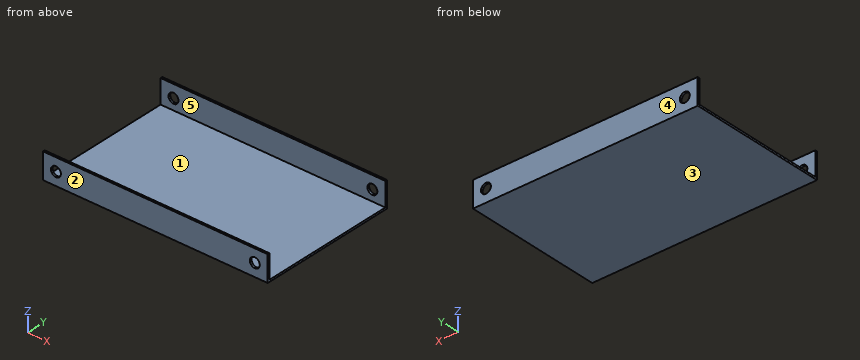
from build123d import *

# Parameters (mm, degrees)
SKETCH3_W               = 287.02
SKETCH3_H               = 177.8
BOSS_EXTRUDE1_DEPTH     = 33.02
SKETCH4_W               = 281.94
SKETCH4_H               = 172.72
CUT_EXTRUDE1_DEPTH      = 30.48
CUT_EXTRUDE2_DEPTH      = 300.87064011
CUT_EXTRUDE2_DEPTH_BACK = 300.87064011
SKETCH5_W               = 30.48
SKETCH5_H               = 172.72
CUT_EXTRUDE3_DEPTH      = 229.913756904
CUT_EXTRUDE3_DEPTH_BACK = 229.913756904
SKETCH6_R               = 6.35


with BuildPart() as part:
    # Sketch3 → Boss-Extrude1 (new body)
    with BuildSketch(Plane.XY):
        Rectangle(SKETCH3_W, SKETCH3_H)
    extrude(amount=BOSS_EXTRUDE1_DEPTH)

    # Sketch4 → Cut-Extrude1 (cut)
    with BuildSketch(Plane.XY.offset(33.02)):
        Rectangle(SKETCH4_W, SKETCH4_H)
    extrude(amount=-CUT_EXTRUDE1_DEPTH, mode=Mode.SUBTRACT)

    # Sketch5 → Cut-Extrude2 (cut, two sides: drawn at the far end of the back side and taken through both)
    with BuildSketch(Plane(origin=(-140.97, 0, 0), x_dir=(0, 0, -1), z_dir=(1, 0, 0)).offset(-CUT_EXTRUDE2_DEPTH_BACK)):
        with Locations((-17.78, 0)):
            Rectangle(SKETCH5_W, SKETCH5_H)
    extrude(amount=CUT_EXTRUDE2_DEPTH + CUT_EXTRUDE2_DEPTH_BACK, mode=Mode.SUBTRACT)

    # Sketch6 → Cut-Extrude3 (cut, two sides: drawn at the far end of the back side and taken through both)
    with BuildSketch(Plane(origin=(0, -86.36, 0), x_dir=(1, 0, 0), z_dir=(0, 1, 0)).offset(-CUT_EXTRUDE3_DEPTH_BACK)):
        with Locations(Location((127, -16.51, 0), (0, 0, 270))):
            Circle(SKETCH6_R)
        with Locations(Location((-127, -16.51, 0), (0, 0, 270))):
            Circle(SKETCH6_R)
    extrude(amount=CUT_EXTRUDE3_DEPTH + CUT_EXTRUDE3_DEPTH_BACK, mode=Mode.SUBTRACT)


solid = part.part
Check sheet for the modelled part. Datum: model origin and axes. Units: mm. Face numbers are marked on the shaded views. A direction names the side the tool comes from. Round coordinates to 2 decimals unless told otherwise and drop trailing zeros. Order: outer loops, then holes, each group sorted by start corner. A loop starts at its lowest first (then second) coordinate and runs counter-clockwise, first axis right, second up.
(1) Cross-section at D-D, the plane y = -61. Enter the section's corners in (x, z).
(2) Access from +Z, -Z, +X, -X, +Y, -Y to the whole of each face (thin tool, end or side, straight path). Record for the marked faces 4 and 5.
(3) Cross-section at B-B, the plane x = 127. Enter the section's corners in (y, z).
(4) Scan lines: probe 1 along X at (y, z) = (87, 16.51); probe 2 along Y at (x, z) = (85.5, 20); probe 3 along Z at (x, y) = (127, 88.35). Record each from-to range of solid material in increasing order.
(5) Cross-section at C-C, the plane x = -14.5. Enter the section's corners in (y, z), and give its area (3 significant figures).
(6) Draft check along Y on the marked faces 1, 2 and 3. Enter one of: pulls with the +Y half, pulls with the -Y half, needs draft (parallel to the pull), parting line crosses it, or undercut.
(7) Go/stop test with flat-tipped pins: P1, Ø1, axis at x = -85, y = -20, coming from the +Z side; P2, Ø11.5, axis at x = 127, z = 16.51, coming from the +Y side. Record where each tip stops, or that it passes through.
(8) Cross-section at A-A, the plane z = 27. Enter the section's corners in (x, y), and give its area (3 significant figures).
Check sheet entries:
1. outline: (-143.51, 0) - (143.51, 0) - (143.51, 2.54) - (-143.51, 2.54) - close
2. face 4: +Z, -Z, +X, -X, +Y
2. face 5: +Z, +X, -X
3. outline: (-88.9, 0) - (88.9, 0) - (88.9, 10.16) - (86.36, 10.16) - (86.36, 2.54) - (-86.36, 2.54) - (-86.36, 10.16) - (-88.9, 10.16) - close; (-88.9, 22.86) - (-86.36, 22.86) - (-86.36, 33.02) - (-88.9, 33.02) - close; (86.36, 22.86) - (88.9, 22.86) - (88.9, 33.02) - (86.36, 33.02) - close
4. probe 1: x = -143.51 to -133.35, -120.65 to 120.65, 133.35 to 143.51
4. probe 2: y = -88.9 to -86.36, 86.36 to 88.9
4. probe 3: z = 0 to 10.16, 22.86 to 33.02
5. outline: (-88.9, 0) - (88.9, 0) - (88.9, 33.02) - (86.36, 33.02) - (86.36, 2.54) - (-86.36, 2.54) - (-86.36, 33.02) - (-88.9, 33.02) - close
5. area: 606 mm2
6. face 1: undercut
6. face 2: pulls with the -Y half
6. face 3: needs draft
7. P1: stops at z = 2.54
7. P2: passes through
8. outline: (-143.51, -88.9) - (143.51, -88.9) - (143.51, -86.36) - (-143.51, -86.36) - close; (-143.51, 86.36) - (143.51, 86.36) - (143.51, 88.9) - (-143.51, 88.9) - close
8. area: 1,460 mm2
